Here's how the part is built. I have some questions about the finished solid (model axes, mm). A direction names the side the tool comes from. Coordinates: 2 decimals unless noted, no trailing zeros. Order: outer loops, then holes, each group sorted by start corner. A loop starts at its lowest first (then second) coordinate and runs counter-clockwise, first axis right, second up. Notation, with made-up numbers: (70.5, -38.75) - (103.5, -38.75) arc R28 cw to (103.5, -13.75) - close; hole circle Ø9 at (10, 49). An arc over 180 degrees is marked (long way). Answer in a Markdown table with one row per item. Add a question column.
Item 1: If I drill on line 1 along Y through (x, z) = (0, 1.75); line 2 along Y through (x, z) = (0.5, 3.5); line 3 along X through (y, z) = (-6, 4.25), over which ranges is the centre line in solid material (lowest first)? Write a range as from..to.
Item 2: On a 3-axis mill with a long thin cutter (end or side, diameter ignored), from which of +Z, -Z, +X, -X, +Y, -Y can I reach the whole of each face in a straight line? I mean faces 4 (the flat face through (0, -3.874, 3)), 5 (the cylindrical face through (7.38, -0.059, 4.526)). Say none if no direction works.
Item 3: I want a section at D-D (y = -3). Please give me the cut outline in (x, z).
Item 4: Will these pins go through, and if not, where does the flat tip stop? pin 1 Ø1 at (y, z) = (9, 1.5) entering from -X; pin 2 Ø2 at (y, z) = (-6, 5) entering from +X; pin 3 Ø2 at (y, z) = (-4, 4.5) entering from +X.
Item 5: Thinking about a two-plate mould opening in Y: for faces 1 (the cylindrical face through (-7.48, -0.82, 2.1)), 2 (the cylindrical face through (10.48, 3.3, 3.13)), 3 (the flat face through (5, 0, 0)), which applies, +Y half, -Y half, draft (parallel to the pull), parting line (faces both ways), or undercut?
Item 6: I want a section at A-A (x = 0). Please give me the cut outline in (y, z).
Item 7: I want a section at B-B (y = 0). Please give me the cut outline in (x, z).
```python
from build123d import *

# Parameters (mm, degrees)
SKETCH1_R                           = 10.9855
SKETCH1_W                           = 7.747
SKETCH1_H                           = 7.747
BOSS_EXTRUDE1_DEPTH                 = 6.35
F_6_32_TAPPED_HOLE1_D               = 2.7051
F_6_32_TAPPED_HOLE1_DEPTH           = 7.112
F_6_32_TAPPED_HOLE1_ON_FACE_2_D     = 2.7051
F_6_32_TAPPED_HOLE1_ON_FACE_2_DEPTH = 7.112
F_6_32_TAPPED_HOLE2_D               = 2.7051
F_6_CLEARANCE_HOLE1_D               = 3.7973


with BuildPart() as part:
    # Sketch1 → Boss-Extrude1 (new body)
    with BuildSketch(Plane.XY):
        Circle(SKETCH1_R)
        Rectangle(SKETCH1_W, SKETCH1_H, mode=Mode.SUBTRACT)
    extrude(amount=BOSS_EXTRUDE1_DEPTH)

    # #6-32 Tapped Hole1
    with Locations(Plane(origin=(10.9855, 0, 3.175), x_dir=(0, 0, 1), z_dir=(1, 0, 0))):
        with Locations((0, 0)):
            Hole(F_6_32_TAPPED_HOLE1_D / 2, depth=F_6_32_TAPPED_HOLE1_DEPTH)

    # #6-32 Tapped Hole1 on face 2
    with Locations(Plane(origin=(3.8735, 0, 3.175), x_dir=(0, 0, -1), z_dir=(-1, 0, 0))):
        with Locations((0, 0)):
            Hole(F_6_32_TAPPED_HOLE1_ON_FACE_2_D / 2, depth=F_6_32_TAPPED_HOLE1_ON_FACE_2_DEPTH)

    # #6-32 Tapped Hole2 (through all)
    with Locations(Plane(origin=(-3.8735, 0, 0), x_dir=(0, 0, -1), z_dir=(1, 0, 0))):
        with Locations((-3.175, 0)):
            Hole(F_6_32_TAPPED_HOLE2_D / 2)

    # #6 Clearance Hole1 (through all)
    with Locations(Plane(origin=(0, 0, 0), x_dir=(-1, 0, 0), z_dir=(0, 0, -1))):
        with Locations((0, -7.4295), (0, 7.4295)):
            Hole(F_6_CLEARANCE_HOLE1_D / 2)


solid = part.part
```
Values follow:
| question | item | result |
|---|---|---|
| 1 | line 1 | y = -10.99..-9.33, -5.53..-3.87, 3.87..5.53, 9.33..10.99 |
| 1 | line 2 | y = -10.97..-9.26, -5.6..-3.87, 3.87..5.6, 9.26..10.97 |
| 1 | line 3 | x = -9.2..-1.25, 1.25..9.2 |
| 2 | face 4 | +Z, -Z |
| 2 | face 5 | +X, -X |
| 3 | outline | (-10.57, 0) - (-3.87, 0) - (-3.87, 6.35) - (-10.57, 6.35) - close; (3.87, 0) - (10.57, 0) - (10.57, 6.35) - (3.87, 6.35) - close |
| 4 | pin 1 | stops at x = -6.96 |
| 4 | pin 2 | stops at x = 9.78 |
| 4 | pin 3 | stops at x = 10.57 |
| 5 | face 1 | undercut |
| 5 | face 2 | parting line |
| 5 | face 3 | draft |
| 6 | outline | (-10.99, 0) - (-9.33, 0) - (-9.33, 6.35) - (-10.99, 6.35) - close; (-5.53, 0) - (-3.87, 0) - (-3.87, 6.35) - (-5.53, 6.35) - close; (3.87, 0) - (5.53, 0) - (5.53, 6.35) - (3.87, 6.35) - close; (9.33, 0) - (10.99, 0) - (10.99, 6.35) - (9.33, 6.35) - close |
| 7 | outline | (-10.99, 0) - (-3.87, 0) - (-3.87, 1.82) - (-10.99, 1.82) - close; (-10.99, 4.53) - (-3.87, 4.53) - (-3.87, 6.35) - (-10.99, 6.35) - close; (3.87, 0) - (10.99, 0) - (10.99, 1.82) - (3.87, 1.82) - close; (3.87, 4.53) - (10.99, 4.53) - (10.99, 6.35) - (3.87, 6.35) - close |
